For this review, take the finished solid that the model builds, in its own axes (mm). Face numbers are marked on the shaded views. A direction names the side the tool comes from. Round coordinates to 2 decimals unless told otherwise and drop trailing zeros. Order: outer loops, then holes, each group sorted by start corner. A loop starts at its lowest first (then second) coordinate and runs counter-clockwise, first axis right, second up. Notation, with made-up numbers: (29, -36.5) - (64, -36.5) arc R29 cw to (64, -13.5) - close; hole circle Ø11 at (86.25, 76). An arc over 180 degrees is marked (long way). One line per question, with ' | ' between items.
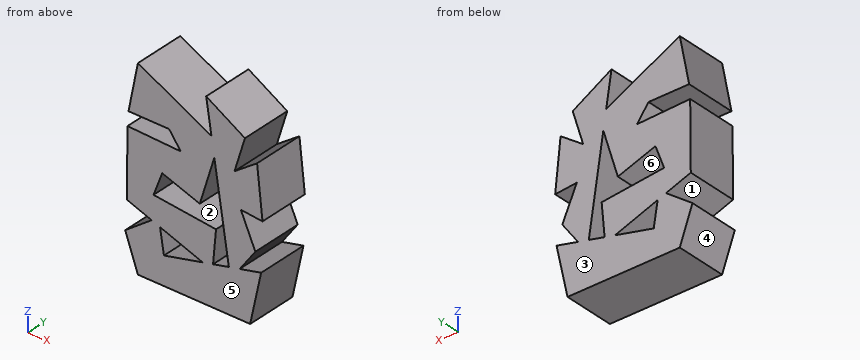
```python
from build123d import *

# Parameters (mm, degrees)
F1_DEPTH = 25


with BuildPart() as f1:
    # F0 (on Front) → F1 (new body)
    with BuildSketch(Plane.XZ):
        Polygon((9.3355238921, 21.5350252004), (5.696185278, 23.3546947243), (7.112640961, 14.2489086105), align=None)
        Polygon((3.1160083599, 39.9415455759), (5.696185278, 23.3546947243), (9.3355238921, 21.5350252004), (7.112640961, 14.2489086105), (14.2324656675, -31.5213909643), (19.5127929437, -30.2641700858), (27.1942447871, -19.5458643138), (20.0996515075, -3.7194623682), (30.695501842, -4.6683449843), (28.0440635979, 20.1124101877), (16.9964041561, 12.1807558462), (22.0953244716, 28.8938842714), align=None)
        Polygon((5.696185278, 23.3546947243), (-30.3102526814, 41.3579158485), (-34.9019161013, 18.1294977665), (-15.0134898722, 18.1294977665), (-9.3480218202, 10.4811154306), (-35.4091748595, 11.3309361041), (-35.6924459338, -21.5287767351), (-23.5665350946, -25.7892328121), (-20.1124101877, -23.2284162194), (-19.4695026466, -27.2287310092), (1.4262612845, -34.5704874846), (6.4912185709, -33.3645451792), (7.9316552728, -17.279677093), (-22.6618722081, -14.1636701301), (-18.4127707034, -2.832734026), (0, -9.0647488832), (7.112640961, 14.2489086105), align=None)
        Polygon((-23.5665350946, -25.7892328121), (-19.4695026466, -27.2287310092), (-20.1124101877, -23.2284162194), align=None)
        Polygon((19.5127929437, -30.2641700858), (14.2324656675, -31.5213909643), (15.0134908035, -36.5422666073), align=None)
        Polygon((6.2320139259, -36.258995533), (6.4912185709, -33.3645451792), (1.4262612845, -34.5704874846), align=None)
        Polygon((15.0134908035, -36.5422666073), (14.2324656675, -31.5213909643), (6.4912185709, -33.3645451792), (6.2320139259, -36.258995533), (1.4262612845, -34.5704874846), (-17.56295003, -39.0917286277), (-19.4695026466, -27.2287310092), (-23.5665350946, -25.7892328121), (-36.5422666073, -35.4091711342), (-30.3102526814, -52.6888519526), (24.6447846293, -52.6888519526), (30.0269778818, -27.7607925236), (19.5127929437, -30.2641700858), align=None)
    extrude(amount=F1_DEPTH)


solid = f1.part
```
(1) Mouldability with a two-part tool opening along X and no side actions: class the marked faces 4, 5 and 6 as released by +X, released by -X, zero draft, split by the parting line, or undercut.
Output values:
face 4: released by -X | face 5: zero draft | face 6: undercut
(2) We need section C-C on z = 7. State the section outline as (x, y) points.
Output values:
outline: (-35.45, -25) - (4.9, -25) - (4.9, 0) - (-35.45, 0) - close; (8.24, -25) - (29.45, -25) - (29.45, 0) - (8.24, 0) - close
(3) We need section A-A on y = -12.75. Give the number of separate pieces and of enclosed holes in the cut face, plus the area to 3 significant figures.
Output values:
separate pieces: 1 | enclosed holes: 2 | area: 4,310 mm^2
(4) We need section D-D on x = 11. State the section outline as (y, z) points, plus the area to 3 significant figures.
Output values:
outline: (-25, -52.69) - (0, -52.69) - (0, -32.29) - (-25, -32.29) - close; (-25, -10.74) - (0, -10.74) - (0, 35.35) - (-25, 35.35) - close | area: 1,660 mm^2
(5) For probe 1 along Z at (x, y) = (-16.5, -24); probe 2 along Z at (x, y) = (-25.5, -17); probe 3 along Z at (x, y) = (-12, -6.75), list the stretches that pass through material, from the lowest coordinate up. Write a range as [from, to].
Output values:
probe 1: [-52.69, -38.84], [-28.27, -14.79], [-3.48, 10.71], [18.13, 34.45] | probe 2: [-52.69, -27.22], [-25.11, 11.01], [18.13, 38.95] | probe 3: [-52.69, -37.77], [-29.85, -15.25], [-5, 10.57], [14.06, 32.2]
(6) We need section B-B on x = -1.5. State the section outline as (y, z) points.
Output values:
outline: (-25, -52.69) - (0, -52.69) - (0, -35.27) - (-25, -35.27) - close; (-25, -33.54) - (0, -33.54) - (0, -16.32) - (-25, -16.32) - close; (-25, -8.56) - (0, -8.56) - (0, 26.95) - (-25, 26.95) - close
(7) Insertion check: pin 1 (2 mm diameter, centred on y = -9, z = 16, fed in from +X); pin 2 (8 mm diameter, centred on x = -29, y = -18, fed in from +Z); pin 3 (5 mm diameter, centred on x = -1, y = -5.5, fed in from +Z); pin 4 (1 mm diameter, centred on x = -21, z = 31.5, fed in from +Y). Each pin has a flat end and moves straight along its axis. Give the tip position at first contact, or say it passes through.
Output values:
pin 1: x = 28.59 | pin 2: z = 41.36 | pin 3: z = 27.95 | pin 4: y = 0
(8) For the marked faces 1, 2 and 3, list the 3-axis set-ups (+Z, -Z, +X, -X, +Y, -Y) from which the entire face can be reached by the end or side of a thin tool; tool diameter is ignored.
Output values:
face 1: -X, +Y, -Y | face 2: +Y, -Y | face 3: +Z, -Z, +X, -X, +Y
